```python
from build123d import *

# Parameters (mm, degrees)
CROQUIS1_W              = 12
CROQUIS1_H              = 12
CROQUIS1_R              = 3.375
SALIENTE_EXTRUIR1_DEPTH = 5
CROQUIS2_W              = 71.4
CROQUIS2_H              = 12
CROQUIS2_R              = 2.1
SALIENTE_EXTRUIR2_DEPTH = 5
CORTAR_EXTRUIR1_REACH   = 84.645
CROQUIS4_R              = 1
CORTAR_EXTRUIR2_START   = -5
CROQUIS5_R              = 2.1
CORTAR_EXTRUIR2_DEPTH   = 3
SALIENTE_EXTRUIR4_START = -1.5
CROQUIS6_R              = 2.1
CROQUIS6_R_2            = 1.1
SALIENTE_EXTRUIR4_DEPTH = 1.5
REDONDEO2_R             = 6
SALIENTE_EXTRUIR5_DEPTH = 5
SALIENTE_EXTRUIR6_DEPTH = 7
CHAFL_N1_SIZE           = 7
CHAFL_N2_SIZE           = 1.5


# Some blends are built 0.0001 mm under size
with BuildPart() as part:
    # Croquis1 → Saliente-Extruir1 (new body)
    # profile 1 of 2: a face of its own
    with BuildSketch(Plane.XY):
        Polygon((25.5, 20), (-6, 20), (-6, 0), (6, 0), (6, 8), (25.5, 8), align=None)
    # profile 2 of 2: a face of its own
    with BuildSketch(Plane.XY):
        with Locations((0, -6)):
            Rectangle(CROQUIS1_W, CROQUIS1_H)
        with Locations((0, -6)):
            Circle(CROQUIS1_R, mode=Mode.SUBTRACT)
    extrude(amount=SALIENTE_EXTRUIR1_DEPTH)

    # Croquis2 → Saliente-Extruir2 (add)
    with BuildSketch(Plane(origin=(25.5, 0, 0), x_dir=(0, 0, -1), z_dir=(1, 0, 0))):
        with Locations((-35.7, 14)):
            Rectangle(CROQUIS2_W, CROQUIS2_H)
        with Locations((-49.4, 14)):
            Circle(CROQUIS2_R, mode=Mode.SUBTRACT)
    extrude(amount=SALIENTE_EXTRUIR2_DEPTH)

    # Croquis4 → Cortar-Extruir1 (cut, up to next)
    with BuildSketch(Plane(origin=(30.5, 0, 0), x_dir=(0, 0, -1), z_dir=(1, 0, 0)), mode=Mode.PRIVATE) as cortar_extruir1_sk1:
        with Locations((-68.4, 14)):
            Circle(CROQUIS4_R)
    cortar_extruir1_tool1 = extrude(cortar_extruir1_sk1.sketch, amount=-CORTAR_EXTRUIR1_REACH, mode=Mode.PRIVATE) & part.part
    # Croquis4 → Cortar-Extruir1 (cut, up to next)
    with BuildSketch(Plane(origin=(30.5, 0, 0), x_dir=(0, 0, -1), z_dir=(1, 0, 0)), mode=Mode.PRIVATE) as cortar_extruir1_sk2:
        with Locations((-64.9, 14)):
            Circle(CROQUIS4_R)
    cortar_extruir1_tool2 = extrude(cortar_extruir1_sk2.sketch, amount=-CORTAR_EXTRUIR1_REACH, mode=Mode.PRIVATE) & part.part
    # Croquis4 → Cortar-Extruir1 (cut, up to next)
    with BuildSketch(Plane(origin=(30.5, 0, 0), x_dir=(0, 0, -1), z_dir=(1, 0, 0)), mode=Mode.PRIVATE) as cortar_extruir1_sk3:
        with Locations((-61.4, 14)):
            Circle(CROQUIS4_R)
    cortar_extruir1_tool3 = extrude(cortar_extruir1_sk3.sketch, amount=-CORTAR_EXTRUIR1_REACH, mode=Mode.PRIVATE) & part.part
    # Croquis4 → Cortar-Extruir1 (cut, up to next)
    with BuildSketch(Plane(origin=(30.5, 0, 0), x_dir=(0, 0, -1), z_dir=(1, 0, 0)), mode=Mode.PRIVATE) as cortar_extruir1_sk4:
        with Locations((-57.9, 14)):
            Circle(CROQUIS4_R)
    cortar_extruir1_tool4 = extrude(cortar_extruir1_sk4.sketch, amount=-CORTAR_EXTRUIR1_REACH, mode=Mode.PRIVATE) & part.part
    # Croquis4 → Cortar-Extruir1 (cut, up to next)
    with BuildSketch(Plane(origin=(30.5, 0, 0), x_dir=(0, 0, -1), z_dir=(1, 0, 0)), mode=Mode.PRIVATE) as cortar_extruir1_sk5:
        with Locations((-40.9, 14)):
            Circle(CROQUIS4_R)
    cortar_extruir1_tool5 = extrude(cortar_extruir1_sk5.sketch, amount=-CORTAR_EXTRUIR1_REACH, mode=Mode.PRIVATE) & part.part
    # Croquis4 → Cortar-Extruir1 (cut, up to next)
    with BuildSketch(Plane(origin=(30.5, 0, 0), x_dir=(0, 0, -1), z_dir=(1, 0, 0)), mode=Mode.PRIVATE) as cortar_extruir1_sk6:
        with Locations((-37.4, 14)):
            Circle(CROQUIS4_R)
    cortar_extruir1_tool6 = extrude(cortar_extruir1_sk6.sketch, amount=-CORTAR_EXTRUIR1_REACH, mode=Mode.PRIVATE) & part.part
    # Croquis4 → Cortar-Extruir1 (cut, up to next)
    with BuildSketch(Plane(origin=(30.5, 0, 0), x_dir=(0, 0, -1), z_dir=(1, 0, 0)), mode=Mode.PRIVATE) as cortar_extruir1_sk7:
        with Locations((-33.9, 14)):
            Circle(CROQUIS4_R)
    cortar_extruir1_tool7 = extrude(cortar_extruir1_sk7.sketch, amount=-CORTAR_EXTRUIR1_REACH, mode=Mode.PRIVATE) & part.part
    # Croquis4 → Cortar-Extruir1 (cut, up to next)
    with BuildSketch(Plane(origin=(30.5, 0, 0), x_dir=(0, 0, -1), z_dir=(1, 0, 0)), mode=Mode.PRIVATE) as cortar_extruir1_sk8:
        with Locations((-30.4, 14)):
            Circle(CROQUIS4_R)
    cortar_extruir1_tool8 = extrude(cortar_extruir1_sk8.sketch, amount=-CORTAR_EXTRUIR1_REACH, mode=Mode.PRIVATE) & part.part
    add(cortar_extruir1_tool1.solids().sort_by_distance((30.5, 14, 68.4))[0], mode=Mode.SUBTRACT)
    add(cortar_extruir1_tool2.solids().sort_by_distance((30.5, 14, 64.9))[0], mode=Mode.SUBTRACT)
    add(cortar_extruir1_tool3.solids().sort_by_distance((30.5, 14, 61.4))[0], mode=Mode.SUBTRACT)
    add(cortar_extruir1_tool4.solids().sort_by_distance((30.5, 14, 57.9))[0], mode=Mode.SUBTRACT)
    add(cortar_extruir1_tool5.solids().sort_by_distance((30.5, 14, 40.9))[0], mode=Mode.SUBTRACT)
    add(cortar_extruir1_tool6.solids().sort_by_distance((30.5, 14, 37.4))[0], mode=Mode.SUBTRACT)
    add(cortar_extruir1_tool7.solids().sort_by_distance((30.5, 14, 33.9))[0], mode=Mode.SUBTRACT)
    add(cortar_extruir1_tool8.solids().sort_by_distance((30.5, 14, 30.4))[0], mode=Mode.SUBTRACT)

    # Croquis5 → Cortar-Extruir2 (cut)
    with BuildSketch(Plane(origin=(30.5, 0, 0), x_dir=(0, 0, -1), z_dir=(1, 0, 0)).offset(CORTAR_EXTRUIR2_START)):
        with Locations((-57.9, 14)):
            Circle(CROQUIS5_R)
        with Locations((-64.9, 14)):
            Circle(CROQUIS5_R)
        with Locations((-40.9, 14)):
            Circle(CROQUIS5_R)
        with Locations((-33.9, 14)):
            Circle(CROQUIS5_R)
    extrude(amount=CORTAR_EXTRUIR2_DEPTH, mode=Mode.SUBTRACT)

    # Croquis6 → Saliente-Extruir4 (add)
    with BuildSketch(Plane(origin=(30.5, 0, 0), x_dir=(0, 0, -1), z_dir=(1, 0, 0)).offset(SALIENTE_EXTRUIR4_START)):
        with Locations((-49.4, 14)):
            Circle(CROQUIS6_R)
        with Locations((-49.4, 14)):
            Circle(CROQUIS6_R_2, mode=Mode.SUBTRACT)
    extrude(amount=SALIENTE_EXTRUIR4_DEPTH)

    # Redondeo2
    # the kernel refuses this fillet: 6 mm, written as the material it takes off along each edge
    with BuildSketch(Plane(origin=(10.5, 20, 71.4), x_dir=(0, 0, -1), z_dir=(1, 0, 0)), Plane(origin=(10.5, 8, 71.4), x_dir=(0, 1, 0), z_dir=(1, 0, 0))) as redondeo2_piece_1:
        with BuildLine():
            CenterArc((REDONDEO2_R, -REDONDEO2_R), REDONDEO2_R, 90, 90)
            Line((0, -REDONDEO2_R), (0, 0))
            Line((0, 0), (REDONDEO2_R, 0))
        make_face()
    extrude(amount=35, mode=Mode.SUBTRACT)

    # Croquis10 → Saliente-Extruir5 (add)
    with BuildSketch(Plane(origin=(0, 0, 0), x_dir=(-1, 0, 0), z_dir=(0, 0, -1))):
        Polygon((-6, 8), (-6, -12), (-30.5, 8), align=None)
    extrude(amount=-SALIENTE_EXTRUIR5_DEPTH)

    # Croquis11 → Saliente-Extruir6 (add)
    with BuildSketch(Plane.XY.offset(5)):
        Polygon((-6, 1), (21.925, 1), (30.5, 8), (25.5, 8), (20.6, 4), (-6, 4), align=None)
    extrude(amount=SALIENTE_EXTRUIR6_DEPTH)

    # Chaflán1
    chafl_n1_edges = [part.edges().sort_by_distance(p)[0] for p in [
        (7.3, 4, 5),
    ]]
    chamfer(chafl_n1_edges, length=CHAFL_N1_SIZE - 0.0001)  # a hair under: the kernel refuses the full size

    # Chaflán2
    chafl_n2_edges = [part.edges().sort_by_distance(p)[0] for p in [
        (12.25, 20, 0),
        (30.5, 14, 71.4),
        (30.5, 14, 71.4),
        (18.25, -2, 0),
        (13.9625, -5.5, 5),
        (30.5, 8, 38.7),
        (-6, -5.5, 5),
        (9.75, 20, 5),
        (-6, 15.49995, 5),
        (30.5, 14, 0),
        (0, -12, 5),
        (30.5, 20, 32.7),
        (0, -12, 0),
        (-6, 4, 0),
    ]]
    chamfer(chafl_n2_edges, length=CHAFL_N2_SIZE)


solid = part.part
```
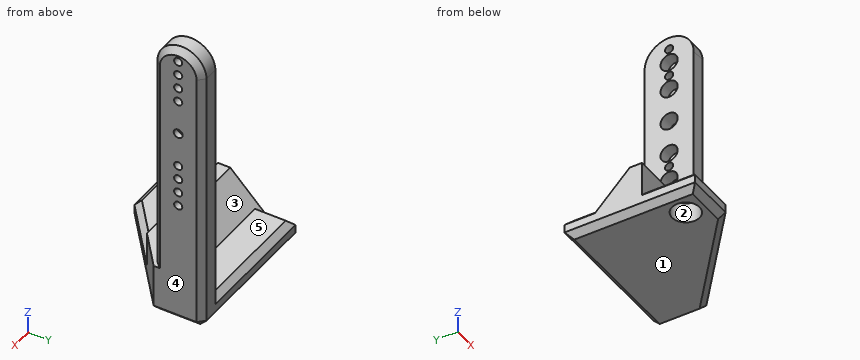
The model under review builds one solid part; all positions refer to its coordinate system, in mm. Face numbers are marked on the shaded views. A direction names the side the tool comes from. Coordinates: 2 decimals unless noted, no trailing zeros. Write each loop counter-clockwise with the first axis right and the second up, starting at its lowest first coordinate (ties: lowest second). Pieces come first, ordered by that corner, then holes. Notation, with made-up numbers: (-19.5, -29) -> (-4.5, -29) arc R20 cw to (-4.5, -4) -> close; hole circle Ø6 at (33, 3.5). An arc over 180 degrees is marked (long way). One line per item, written item: value. Start each with the question number.
Q1. Add section B-B, the plane y = -6. Give the boundary of the cut face in (x, z) (3 decimals).
Q2. Add section D-D, the plane y = 14. Count the separate pieces of the cut face and the enclosed holes in it, then the cut area to 3 significant figures.
Q3. Clearance check with flat-ended pins moving along their axes: P1, Ø1, axis at x = 10.5, y = -7, coming from the -Z side; P2, Ø4.5, axis at y = 15, z = 64.5, coming from the -X side; P3, Ø4, axis at x = -1.5, y = -5, coming from the +Z side; P4, Ø2.5, axis at y = 14, z = 40.9, coming from the -X side. State where each tip first meets the part, or that it passes through.
Q4. To check wall thickness, follow probe 1 along Z at (x, y) = (8.5, -7); probe 2 along X at (y, z) = (15, 23); probe 3 along X at (y, z) = (13, 42). State the ranges of each line that lie inside material, in increasing order.
Q5. For the marked faces 4 and 5, list the 3-axis set-ups (+Z, -Z, +X, -X, +Y, -Y) from which the entire face can be reached by the end or side of a thin tool; tool diameter is ignored.
Q6. Add section A-A, the plane z = 40.9. Give the boundary of the cut face in (x, y).
Q7. The part is to be moulded in two halves that separate along Y. For the marked faces 1, 2 and 3, say which applies: +Y half, -Y half, draft (parallel to the pull), parting line (faces both ways), or undercut.
Response:
1. outline: (-6, 1.5) -> (-4.5, 0) -> (-3.375, 0) -> (-3.375, 5) -> (-4.5, 5) -> (-6, 3.5) -> close; (3.375, 0) -> (10.978, 0) -> (13.35, 1.5) -> (13.35, 3.5) -> (10.978, 5) -> (3.375, 5) -> close
2. separate pieces: 10
2. enclosed holes: 0
2. area: 386 mm²
3. P1: z = 0
3. P2: x = 25.5
3. P3: z = 5
3. P4: x = 28.5
4. probe 1: 0 to 5
4. probe 2: 25.5 to 30.5
4. probe 3: 28.5 to 30.5
5. face 4: +Z, -Z, +X, +Y, -Y
5. face 5: +Z, -X, +Y
6. outline: (25.5, 8) -> (29, 8) -> (30.5, 9.5) -> (30.5, 13) -> (28.5, 13) -> (28.5, 11.9) -> (25.5, 11.9) -> close; (25.5, 16.1) -> (28.5, 16.1) -> (28.5, 15) -> (30.5, 15) -> (30.5, 18.5) -> (29, 20) -> (25.5, 20) -> close
7. face 1: draft
7. face 2: undercut
7. face 3: +Y half
